from build123d import *

# Parameters (mm, degrees)
BOSS_EXTRUDE1_DEPTH = 8
CUT_EXTRUDE2_DEPTH  = 9


with BuildPart() as part:
    # Sketch1 → Boss-Extrude1 (new body)
    with BuildSketch(Plane.XY):
        with BuildLine():
            Line((12.878924965, 0.299989593), (12.889991366, 2.998769855))
            Line((12.889991366, 2.998769855), (12.889991366, 3.3))
            Line((12.889991366, 3.3), (12.589993889, 3.3))
            Line((12.589993889, 3.3), (12.227716247, 3.3))
            ThreePointArc((12.227716247, 3.3), (7.127300009, 5.014869597), (3.3, 8.797302437))
            Line((3.3, 8.797302437), (3.3, 14.423444914))
            Line((3.3, 14.423444914), (3.3, 14.723444914))
            Line((3.3, 14.723444914), (3, 14.723444914))
            Line((3, 14.723444914), (0.3, 14.723444914))
            Line((0.3, 14.723444914), (0.3, 15.615227729))
            Line((0.3, 15.615227729), (3, 15.615227729))
            Line((3, 15.615227729), (3.3, 15.615227729))
            Line((3.3, 15.615227729), (3.3, 15.915227729))
            Line((3.3, 15.915227729), (3.3, 21.541370205))
            ThreePointArc((3.3, 21.541370205), (7.127300009, 25.323803045), (12.227716247, 27.038672642))
            Line((12.227716247, 27.038672642), (12.589994095, 27.038672642))
            Line((12.589994095, 27.038672642), (12.889991573, 27.038672642))
            Line((12.889991573, 27.038672642), (12.889991573, 27.339902808))
            Line((12.889991573, 27.339902808), (12.889991573, 30.038672936))
            Line((12.889991573, 30.038672936), (13.756179426, 30.038672936))
            Line((13.756179426, 30.038672936), (13.756179426, 27.338672642))
            Line((13.756179426, 27.338672642), (13.756179426, 27.038672642))
            Line((13.756179426, 27.038672642), (14.056179426, 27.038672642))
            Line((14.056179426, 27.038672642), (14.40506038, 27.038672642))
            ThreePointArc((14.40506038, 27.038672642), (19.505476619, 25.323803045), (23.332776628, 21.541370205))
            Line((23.332776628, 21.541370205), (23.332776628, 15.915227729))
            Line((23.332776628, 15.915227729), (23.332776628, 15.615227729))
            Line((23.332776628, 15.615227729), (23.632776628, 15.615227729))
            Line((23.632776628, 15.615227729), (26.333196522, 15.615227729))
            Line((26.333196522, 15.615227729), (26.333196522, 14.723444914))
            Line((26.333196522, 14.723444914), (23.633196522, 14.723444914))
            Line((23.633196522, 14.723444914), (23.333196522, 14.723444914))
            Line((23.333196522, 14.723444914), (23.333196522, 14.423444914))
            Line((23.333196522, 14.423444914), (23.333196522, 8.797302437))
            ThreePointArc((23.333196522, 8.797302437), (19.505896514, 5.014869597), (14.405480275, 3.3))
            Line((14.405480275, 3.3), (14.056599321, 3.3))
            Line((14.056599321, 3.3), (13.756599321, 3.3))
            Line((13.756599321, 3.3), (13.756599321, 3))
            Line((13.756599321, 3), (13.756599321, 0.3))
            Line((13.756599321, 0.3), (12.878924965, 0.299989593))
        make_face()
    extrude(amount=BOSS_EXTRUDE1_DEPTH)

    # Sketch2 → Cut-Extrude2 (cut, through all)
    with BuildSketch(Plane.XY.offset(8)):
        with BuildLine():
            Line((12.889991573, 30.038672936), (-3.324020912, 25.076549212))
            Line((-3.324020912, 25.076549212), (0.3, 15.615227729))
            Line((0.3, 15.615227729), (3.3, 15.615227729))
            Line((3.3, 15.615227729), (3.3, 21.541370205))
            ThreePointArc((3.3, 21.541370205), (7.127300009, 25.323803045), (12.227716247, 27.038672642))
            Line((12.227716247, 27.038672642), (12.889991573, 27.038672642))
            Line((12.889991573, 27.038672642), (12.889991573, 30.038672936))
        make_face()
        with BuildLine():
            Line((26.333196522, 15.615227729), (25.678702072, 25.392177395))
            Line((25.678702072, 25.392177395), (13.756179426, 30.038672936))
            Line((13.756179426, 30.038672936), (13.756179426, 27.038672642))
            Line((13.756179426, 27.038672642), (14.40506038, 27.038672642))
            ThreePointArc((14.40506038, 27.038672642), (19.505476619, 25.323803045), (23.332776628, 21.541370205))
            Line((23.332776628, 21.541370205), (23.332776628, 15.615227729))
            Line((23.332776628, 15.615227729), (26.333196522, 15.615227729))
        make_face()
        with BuildLine():
            Line((21.332776628, 20.933212865), (21.332776628, 15.615227729))
            Line((21.332776628, 15.615227729), (23.332776628, 15.615227729))
            Line((23.332776628, 15.615227729), (23.332776628, 21.541370205))
            ThreePointArc((23.332776628, 21.541370205), (19.505476619, 25.323803045), (14.40506038, 27.038672642))
            Line((14.40506038, 27.038672642), (13.756179426, 27.038672642))
            Line((13.756179426, 27.038672642), (13.756179426, 25.038672642))
            Line((13.756179426, 25.038672642), (14.303761373, 25.038672642))
            ThreePointArc((14.303761373, 25.038672642), (18.258523966, 23.739709455), (21.332776628, 20.933212865))
        make_face()
        with BuildLine():
            Line((12.329015255, 25.038672642), (12.889991573, 25.038672642))
            Line((12.889991573, 25.038672642), (12.889991573, 27.038672642))
            Line((12.889991573, 27.038672642), (12.227716247, 27.038672642))
            ThreePointArc((12.227716247, 27.038672642), (7.127300009, 25.323803045), (3.3, 21.541370205))
            Line((3.3, 21.541370205), (3.3, 15.615227729))
            Line((3.3, 15.615227729), (5.3, 15.615227729))
            Line((5.3, 15.615227729), (5.3, 20.933212865))
            ThreePointArc((5.3, 20.933212865), (8.374252661, 23.739709455), (12.329015255, 25.038672642))
        make_face()
        with BuildLine():
            Line((5.3, 9.405459777), (5.3, 14.723444914))
            Line((5.3, 14.723444914), (3.3, 14.723444914))
            Line((3.3, 14.723444914), (3.3, 8.797302437))
            ThreePointArc((3.3, 8.797302437), (7.127300009, 5.014869597), (12.227716247, 3.3))
            Line((12.227716247, 3.3), (12.884961194, 3.3))
            Line((12.884961194, 3.3), (12.888985332, 5.3))
            Line((12.888985332, 5.3), (12.329015255, 5.3))
            ThreePointArc((12.329015255, 5.3), (8.374252661, 6.598963188), (5.3, 9.405459777))
        make_face()
        with BuildLine():
            Line((3.3, 8.797302437), (3.3, 14.723444914))
            Line((3.3, 14.723444914), (0.3, 14.723444914))
            Line((0.3, 14.723444914), (4.782985331, 0.07504351))
            Line((4.782985331, 0.07504351), (12.878924965, 0.299989593))
            Line((12.878924965, 0.299989593), (12.884961194, 3.3))
            Line((12.884961194, 3.3), (12.227716247, 3.3))
            ThreePointArc((12.227716247, 3.3), (7.127300009, 5.014869597), (3.3, 8.797302437))
        make_face()
        with BuildLine():
            Line((13.756599321, 5.3), (13.756599321, 3.3))
            Line((13.756599321, 3.3), (14.405480275, 3.3))
            ThreePointArc((14.405480275, 3.3), (19.505896514, 5.014869597), (23.333196522, 8.797302437))
            Line((23.333196522, 8.797302437), (23.333196522, 14.723444914))
            Line((23.333196522, 14.723444914), (21.333196522, 14.723444914))
            Line((21.333196522, 14.723444914), (21.333196522, 9.405459777))
            ThreePointArc((21.333196522, 9.405459777), (18.258943861, 6.598963188), (14.304181268, 5.3))
            Line((14.304181268, 5.3), (13.756599321, 5.3))
        make_face()
        with BuildLine():
            Line((13.756599321, 0.3), (29.080472483, 10.031605851))
            Line((29.080472483, 10.031605851), (26.333196522, 14.723444914))
            Line((26.333196522, 14.723444914), (23.333196522, 14.723444914))
            Line((23.333196522, 14.723444914), (23.333196522, 8.797302437))
            ThreePointArc((23.333196522, 8.797302437), (19.505896514, 5.014869597), (14.405480275, 3.3))
            Line((14.405480275, 3.3), (13.756599321, 3.3))
            Line((13.756599321, 3.3), (13.756599321, 0.3))
        make_face()
    extrude(amount=-CUT_EXTRUDE2_DEPTH, mode=Mode.SUBTRACT)


solid = part.part
Design review of the part built by this model. Coordinates are the model's own, in mm. A direction names the side the tool comes from. Round coordinates to 2 decimals unless told otherwise and drop trailing zeros. Write each loop counter-clockwise with the first axis right and the second up, starting at its lowest first coordinate (ties: lowest second). Pieces come first, ordered by that corner, then holes. Notation, with made-up numbers: M 14.25,-4.75 L 30.25,-4.75 A14 ccw 30.25,5.25 Z; hole C -18.5,-9.75 d1. An arc over 180 degrees is marked long. One line per item, written item: value. Start each with the question number.
1. Clearance check with flat-ended pins moving along their axes: P1, Ø2, axis at y = 19.5, z = 6, coming from the -X side; P2, Ø4, axis at y = 6, z = 4.5, coming from the +X side; P3, Ø4, axis at y = 2.5, z = 4.5, coming from the +X side. State where each tip first meets the part, or that it passes through.
2. For faces 1 (the face through (21.333, 12, 4)), 2 (the face through (12.89, 28, 4)), 3 (the face through (13.3, 30.039, 3.9)), 4 (the face through (24, 15.615, 4)), 5 (the face through (5.3, 12, 4)), list the 3-axis set-ups (+Z, -Z, +X, -X, +Y, -Y) from which the entire face can be reached by the end or side of a thin tool; tool diameter is ignored.
3. Take a section at B-B on x = 3. State the section outline as (y, z) points.
4. Take a section at C-C on y = 26.75. State the section outline as (x, z) points.
5. Take a section at A-A on z = 7.25. State the section outline as (x, y) points (3 decimals).
6. To check wall thickness, follow probe 1 along X at (y, z) = (16.75, 5.5); probe 2 along Y at (x, z) = (24, 2.25); probe 3 along Y at (x, z) = (12.75, 6.5). State the ranges of each line that lie inside material, in increasing order. Write a range as from..to.
Computed:
1. P1: stops at x = 5.3
1. P2: stops at x = 20.12
1. P3: stops at x = 13.76
2. face 1: +Z, -Z, +X, -Y
2. face 2: +Z, -Z, -X, +Y
2. face 3: +Z, -Z, +X, -X, +Y
2. face 4: +Z, -Z, +X, +Y
2. face 5: +Z, -Z, -X, -Y
3. outline: M 14.72,0 L 15.62,0 L 15.62,8 L 14.72,8 Z
4. outline: M 12.89,0 L 13.76,0 L 13.76,8 L 12.89,8 Z
5. outline: M 0.3,14.723 L 5.3,14.723 L 5.3,9.405 A9.925 ccw 12.329,5.3 L 12.889,5.3 L 12.885,3.3 L 12.89,3.3 L 12.89,2.999 L 12.879,0.3 L 13.757,0.3 L 13.757,5.3 L 14.304,5.3 A9.925 ccw 21.333,9.405 L 21.333,14.723 L 26.333,14.723 L 26.333,15.615 L 21.333,15.615 L 21.333,20.933 A9.925 ccw 14.304,25.039 L 13.756,25.039 L 13.756,30.039 L 12.89,30.039 L 12.89,25.039 L 12.329,25.039 A9.925 ccw 5.3,20.933 L 5.3,15.615 L 0.3,15.615 Z
6. probe 1: x = 5.3..21.33
6. probe 2: y = 14.72..15.62
6. probe 3: y = 5.3..25.04
